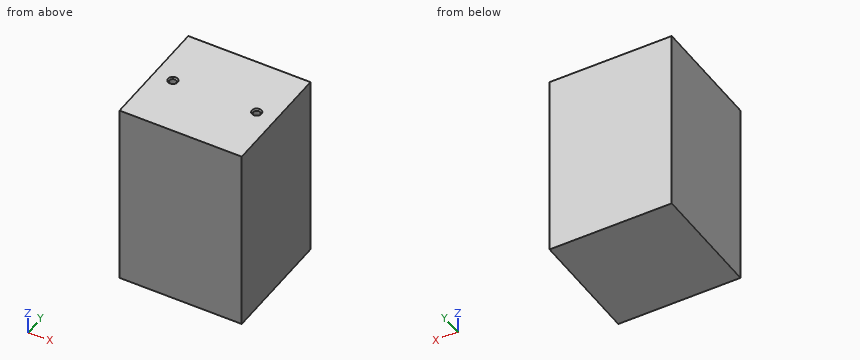
from build123d import *

# Parameters (mm, degrees)
SKETCH4_W                       = 88.626489964
SKETCH4_H                       = 130.535595586
BOSS_EXTRUDE3_DEPTH             = 42.25
SHELL1_T                        = 1
SKETCH5_W                       = 88.626489964
SKETCH5_H                       = 84.5
BOSS_EXTRUDE4_DEPTH             = 5.5
M6X1_0_TAPPED_HOLE1_D           = 5
M6X1_0_TAPPED_HOLE1_DEPTH       = 6.5
M6X1_0_TAPPED_HOLE1_CSINK_D     = 7
M6X1_0_TAPPED_HOLE1_CSINK_ANGLE = 90


with BuildPart() as part:
    # Sketch4 → Boss-Extrude3 (new body, symmetric)
    with BuildSketch(Plane(origin=(0, 0, 0), x_dir=(1, 0, 0), z_dir=(0, 1, 0))):
        Rectangle(SKETCH4_W, SKETCH4_H)
    extrude(amount=BOSS_EXTRUDE3_DEPTH, both=True)

    # Shell1 (no face opened: a closed hollow body)
    add(offset(amount=-SHELL1_T, mode=Mode.PRIVATE), mode=Mode.SUBTRACT)

    # Sketch5 → Boss-Extrude4 (add)
    with BuildSketch(Plane.XY.offset(65.267797793)):
        Rectangle(SKETCH5_W, SKETCH5_H)
    extrude(amount=BOSS_EXTRUDE4_DEPTH)

    # M6x1.0 Tapped Hole1
    with Locations(Plane.XY.offset(70.767797793)):
        with Locations((30.265999315, 0), (-30.578112918, 0)):
            CounterSinkHole(M6X1_0_TAPPED_HOLE1_D / 2, M6X1_0_TAPPED_HOLE1_CSINK_D / 2, depth=M6X1_0_TAPPED_HOLE1_DEPTH, counter_sink_angle=M6X1_0_TAPPED_HOLE1_CSINK_ANGLE)


solid = part.part
Can you work these out from the model? Positions are in its coordinate system, mm. Coordinates: 2 decimals unless noted, no trailing zeros. Write each loop counter-clockwise with the first axis right and the second up, starting at its lowest first coordinate (ties: lowest second). Pieces come first, ordered by that corner, then holes. Notation, with made-up numbers: (-38, -29) -> (-21, -29) arc R21 ccw to (-21, -13) -> close; hole circle Ø9 at (50, -11.75). An arc over 180 degrees is marked (long way). Write item = value, one per line.
(1) Imagine slicing it at B-B (z = -46). Please give me the cut outline in (x, y).
Verdict:
outline = (-44.31, -42.25) -> (44.31, -42.25) -> (44.31, 42.25) -> (-44.31, 42.25) -> close; hole (-43.31, -41.25) -> (43.31, -41.25) -> (43.31, 41.25) -> (-43.31, 41.25) -> close
(2) If I drill on probe 1 along X at (y, z) = (0, 68); probe 2 along Z at (x, y) = (-22.5, -17); probe 3 along Y at (x, z) = (-35, -29), over which ranges is the centre line in solid material (lowest first)?
Verdict:
probe_1 = -44.31 to -33.08, -28.08 to 27.77, 32.77 to 44.31
probe_2 = -65.27 to -64.27, 64.27 to 70.77
probe_3 = -42.25 to -41.25, 41.25 to 42.25
(3) For pin 1 (4 mm diameter, centred on x = 30.266, y = 0, fed in from +Z), with a flat end and sliding along its axis, tell me the tip position at first contact or that it passes through.
Verdict:
pin_1 = -64.27
(4) Imagine slicing it at C-C (x = -37). Please give me the cut outline in (y, z), and give its area (3 significant figures).
Verdict:
outline = (-42.25, -65.27) -> (42.25, -65.27) -> (42.25, 70.77) -> (-42.25, 70.77) -> close; hole (-41.25, -64.27) -> (41.25, -64.27) -> (41.25, 64.27) -> (-41.25, 64.27) -> close
area = 891 mm^2
(5) Imagine slicing it at A-A (y = 0). Please give me the cut outline in (x, z).
Verdict:
outline = (-44.31, -65.27) -> (44.31, -65.27) -> (44.31, 70.77) -> (33.77, 70.77) -> (32.77, 69.77) -> (32.77, 64.27) -> (43.31, 64.27) -> (43.31, -64.27) -> (-43.31, -64.27) -> (-43.31, 64.27) -> (-33.08, 64.27) -> (-33.08, 69.77) -> (-34.08, 70.77) -> (-44.31, 70.77) -> close; (-28.08, 64.27) -> (27.77, 64.27) -> (27.77, 69.77) -> (26.77, 70.77) -> (-27.08, 70.77) -> (-28.08, 69.77) -> close
